Could you check a few things on this model? Use its own coordinates, in mm. A direction names the side the tool comes from. Round coordinates to 2 decimals unless told otherwise and drop trailing zeros. Order: outer loops, then holes, each group sorted by start corner. A loop starts at its lowest first (then second) coordinate and runs counter-clockwise, first axis right, second up. Notation, with made-up numbers: M 78,14.5 L 94,14.5 A33 cw 94,47.5 Z; hole C 16,84.5 d10. An arc over 180 degrees is marked long. Write each question's results on one line, items separated by ' | '. Start each with the question number.
1. Please list where these lines run through material, in increasing order: L1, parallel to Z at x = 32, y = 0; L2, parallel to Y at x = 17, z = 4.5.
2. I'm going to push flat-ended pins straight in: pin 1 (8 mm diameter, centred on x = 37.5, y = -13.5, fed in from +Z); pin 2 (8 mm diameter, centred on x = 7.5, z = 7, fed in from -Y); pin 3 (3 mm diameter, centred on x = 25.5, z = -0.5, fed in from +Y). Where does each tip first touch, or does it pass through?
3. Suppose I cut it at C-C on z = -7. Write out the boundary of the cut face in (x, y).
4. Suppose I cut it at B-B on x = 3. Write out the boundary of the cut face in (y, z), and give its area (3 significant figures).
5. For faces 4 (the cylindrical face through (50.07, 18.89, -8.58)), 5 (the flat face through (45, 14, 0)), which set-ups out of +Z, -Z, +X, -X, +Y, -Y let a thin tool reach every point of the face, with its end or its side?
6. We'd pull the mould along Z, two halves only. Please class faces 1 (the cylindrical face through (27.12, 5.57, -2.23)), 2 (the cylindrical face through (22.18, -11.99, -0.53)), 3 (the flat face through (45, -16, 0)): released by +Z, released by -Z, zero draft, split by the parting line, or undercut.
7. Suppose I cut it at D-D on y = 13.5. Write out the boundary of the cut face in (x, z), and give its area (3 significant figures).
8. Suppose I cut it at A-A on z = 2.5. Write out the boundary of the cut face in (x, y).
Autodesk Inventor part; units mm, degrees
ref_plane "YZ Plane" through (0, 0, 0) normal (1, 0, 0) x (0, 1, 0)
ref_plane "XZ Plane" through (0, 0, 0) normal (0, 1, 0) x (-1, 0, 0)
ref_plane "XY Plane" through (0, 0, 0) normal (0, 0, 1) x (1, 0, 0)
sketch "Sketch1" plane through (0, 0, 0) normal (1, 0, 0) x (0, 1, 0)
  circle A0 centre (0, 0) radius 6
  circle A1 centre (0, 0) radius 12
  dimension "d0" = 12
  dimension "d1" = 24
extrude "Extrusion1" add sketch "Sketch1" along normal blind 45
sketch "Sketch2" plane through (45, 0, 0) normal (1, 0, 0) x (0, 0, -1)
  circle A0 centre (0, 0) radius 6
  circle A1 centre (0, 0) radius 12
  line L0 (12, -22.5) -> (-12, -22.5)
  line L1 (-12, -22.5) -> (-12, 22.5)
  line L2 (-12, 22.5) -> (12, 22.5)
  line L3 (12, 22.5) -> (12, -22.5)
  line L4 (0, 0) -> (3.4418, 0)
  point P0 (12, 0)
  dimension "d4" = 45
extrude "Extrusion2" add sketch "Sketch2" along normal blind 10
fillet "Fillet1" radius 12 4 edges at (50, -22.5, -12) (50, -22.5, 12) (50, 22.5, -12) (50, 22.5, 12)
thread "Thread1"
properties part number "Rotator" material "Steel, Alloy"
Filled sheet:
1) L1: z = -12 to -6, 6 to 12 | L2: y = -11.12 to -3.97, 3.97 to 11.12
2) pin 1: stops at z = 7.33 | pin 2: stops at y = -11.62 | pin 3: stops at y = 12
3) outline: M 0,-9.75 L 45,-9.75 L 45,-20.25 L 55,-20.25 L 55,20.25 L 45,20.25 L 45,9.75 L 0,9.75 Z
4) outline: C 0,0 d24; hole C 0,0 d12 | area: 339 mm^2
5) face 4: -Z, +X, -X, +Y | face 5: -X, +Y
6) face 1: undercut | face 2: split by the parting line | face 3: zero draft
7) outline: M 45,-11.62 L 55,-11.62 L 55,11.62 L 45,11.62 Z | area: 232 mm^2
8) outline: M 0,-11.74 L 45,-11.74 L 45,-22.24 L 55,-22.24 L 55,-5.45 L 0,-5.45 Z; M 0,5.45 L 55,5.45 L 55,22.24 L 45,22.24 L 45,11.74 L 0,11.74 Z
